Read the model definition and answer for the solid it produces. Units are mm, in the model's axes. A direction names the side the tool comes from. Round coordinates to 2 decimals unless told otherwise and drop trailing zeros. Loops run counter-clockwise (first coordinate to the right, second up) from the corner with the lowest first, then second, coordinate; pieces in that order, holes last. Notation, with made-up numbers: (31, -29.75) - (68, -29.75) arc R14 ccw to (68, -5.75) - close; hole circle Ø6 at (16, 74.5). An arc over 180 degrees is marked (long way). Use one line per item in the form item = value. Start each with the question number.
```python
from build123d import *

# Parameters (mm, degrees)
SKETCH2_W           = 33.15
SKETCH2_H           = 33
BOSS_EXTRUDE1_DEPTH = 7.5
SKETCH3_R           = 1.175
CUT_EXTRUDE1_DEPTH  = 4.5
SKETCH4_W           = 5.3
SKETCH4_H           = 7
CUT_EXTRUDE2_DEPTH  = 3.4
SKETCH5_W           = 17.312690108
SKETCH5_H           = 1.808425299
CUT_EXTRUDE3_DEPTH  = 2
SKETCH6_W           = 5.3
SKETCH6_H           = 3.3
CUT_EXTRUDE4_DEPTH  = 25.560753755
CHAMFER3_SIZE       = 11
CHAMFER3_SIZE2      = 6.350852961
SKETCH7_W           = 3
SKETCH7_H           = 33
SKETCH7_H_2         = 30
BOSS_EXTRUDE2_DEPTH = 52.5
SKETCH8_W           = 33.15
SKETCH8_H           = 60
BOSS_EXTRUDE3_DEPTH = 1
SKETCH9_W           = 3
SKETCH9_H           = 34
CUT_EXTRUDE5_DEPTH  = 60
SKETCH10_R          = 0.75
CUT_EXTRUDE6_DEPTH  = 2
SKETCH11_R          = 0.8
CUT_EXTRUDE7_DEPTH  = 2
SKETCH12_R          = 0.8
CUT_EXTRUDE9_DEPTH  = 5.8


with BuildPart() as part:
    # Sketch2 → Boss-Extrude1 (new body)
    with BuildSketch(Plane.XY):
        Rectangle(SKETCH2_W, SKETCH2_H)
    extrude(amount=BOSS_EXTRUDE1_DEPTH)

    # Sketch3 → Cut-Extrude1 (cut)
    with BuildSketch(Plane.XY):
        with Locations((10.325, 10.25)):
            Circle(SKETCH3_R)
        with Locations((-10.325, 10.25)):
            Circle(SKETCH3_R)
        with Locations((10.325, -10.25)):
            Circle(SKETCH3_R)
        with Locations((-10.325, -10.25)):
            Circle(SKETCH3_R)
    extrude(amount=CUT_EXTRUDE1_DEPTH, mode=Mode.SUBTRACT)

    # Sketch4 → Cut-Extrude2 (cut)
    with BuildSketch(Plane.XY):
        with Locations((9.775, 0)):
            Rectangle(SKETCH4_W, SKETCH4_H)
        with Locations((-9.775, 0)):
            Rectangle(SKETCH4_W, SKETCH4_H)
    extrude(amount=CUT_EXTRUDE2_DEPTH, mode=Mode.SUBTRACT)

    # Sketch5 → Cut-Extrude3 (cut)
    with BuildSketch(Plane.XY):
        with Locations((-0.109621432, -11.80915301)):
            Rectangle(SKETCH5_W, SKETCH5_H)
    extrude(amount=CUT_EXTRUDE3_DEPTH, mode=Mode.SUBTRACT)

    # Sketch6 → Cut-Extrude4 (cut, through all)
    with BuildSketch(Plane.XY):
        Rectangle(SKETCH6_W, SKETCH6_H)
    extrude(amount=CUT_EXTRUDE4_DEPTH, mode=Mode.SUBTRACT)

    # Chamfer3
    chamfer3_edges = [part.edges().sort_by_distance(p)[0] for p in [
        (2.65, 0, 7.5),
        (0, 1.65, 7.5),
        (-2.65, 0, 7.5),
        (0, -1.65, 7.5),
    ]]
    chamfer3_side = [part.faces().sort_by_distance(p)[0] for p in [
        (-16.107247662, 0, 7.5),
    ]]
    chamfer(chamfer3_edges, length=CHAMFER3_SIZE, length2=CHAMFER3_SIZE2, reference=chamfer3_side[0])

    # Sketch7 → Boss-Extrude2 (add)
    with BuildSketch(Plane.XY):
        with Locations((15.075, 0)):
            Rectangle(SKETCH7_W, SKETCH7_H)
        Polygon((-13.575, 13.5), (13.575, 13.5), (13.575, 16.5), (-16.575, 16.5), (-16.575, 13.5), align=None)
        with Locations((-15.075, -1.5)):
            Rectangle(SKETCH7_W, SKETCH7_H_2)
    extrude(amount=-BOSS_EXTRUDE2_DEPTH)

    # Sketch8 → Boss-Extrude3 (add)
    with BuildSketch(Plane(origin=(0, 16.5, 0), x_dir=(1, 0, 0), z_dir=(0, 1, 0))):
        with Locations((0, 22.5)):
            Rectangle(SKETCH8_W, SKETCH8_H)
    extrude(amount=BOSS_EXTRUDE3_DEPTH)

    # Sketch9 → Cut-Extrude5 (cut)
    with BuildSketch(Plane(origin=(0, 0, -52.5), x_dir=(-1, 0, 0), z_dir=(0, 0, -1))):
        with Locations((15.075, 0.5)):
            Rectangle(SKETCH9_W, SKETCH9_H)
    extrude(amount=-CUT_EXTRUDE5_DEPTH, mode=Mode.SUBTRACT)

    # Sketch10 → Cut-Extrude6 (cut)
    with BuildSketch(Plane.ZY.offset(13.575)):
        with Locations((-50, 15.5)):
            Circle(SKETCH10_R)
        with Locations(Location((5, 15.5, 0), (0, 0, 180))):
            Circle(SKETCH10_R)
        with Locations((5, -14.5)):
            Circle(SKETCH10_R)
    extrude(amount=-CUT_EXTRUDE6_DEPTH, mode=Mode.SUBTRACT)

    # Sketch11 → Cut-Extrude7 (cut)
    with BuildSketch(Plane(origin=(0, -16.5, 0), x_dir=(-1, 0, 0), z_dir=(0, -1, 0))):
        with Locations(Location((-15.075, 49.5, 0), (0, 0, 90))):
            Circle(SKETCH11_R)
        with Locations(Location((-15.075, -4.5, 0), (0, 0, 270))):
            Circle(SKETCH11_R)
        with Locations(Location((12.075, -4.5, 0), (0, 0, 90))):
            Circle(SKETCH11_R)
    extrude(amount=-CUT_EXTRUDE7_DEPTH, mode=Mode.SUBTRACT)

    # Sketch12 → Cut-Extrude9 (cut)
    with BuildSketch(Plane(origin=(0, 0, -52.5), x_dir=(-1, 0, 0), z_dir=(0, 0, -1))):
        with Locations((-14.575, 15.5)):
            Circle(SKETCH12_R)
        with Locations((-15.075, -14.5)):
            Circle(SKETCH12_R)
    extrude(amount=-CUT_EXTRUDE9_DEPTH, mode=Mode.SUBTRACT)


solid = part.part
```
1) Straight lines are drawn through the part: line 1 (Y direction, x = -12, z = -50); line 2 (X direction, y = -14.5, z = -48.9) (3 decimals); line 3 (Y direction, x = 6, z = -19.5). For each, find the intervals that lie inside material, in ascending order. Write a range as from..to.
2) A cutting plane is placed at D-D on y = 7.5. Write down the section's boundary in (x, z) (3 decimals), plus the area to 3 significant figures.
3) A cutting plane is placed at A-A on x = -1. Write down the section's boundary in (y, z), plus the area to 3 significant figures.
4) For faces 5 (the flat face through (10, 10, 4.5)), 6 (the flat face through (0.23, 8.3, 4.99)), 7 (the cylindrical face through (-12.589, -13.868, 5.403)), determine the directions among +Z, -Z, +X, -X, +Y, -Y from which every point of the face is accessible in a straight line to the end or side of a thin tool.
5) A cutting plane is placed at C-C on z = -41.5. Write down the section's boundary in (x, y) (3 decimals), plus the area to 3 significant figures.
6) Determine the mould class of faces 1 (the flat face through (15, -14.5, 4)), 2 (the flat face through (0.23, -8.3, 4.99)), 3 (the flat face through (15, -14, -46.7)), 4 (the flat face through (16.575, 0, -22)) for opening direction Z: +Z half, -Z half, draft (parallel to the pull), parting line (faces both ways), or undercut.
7) A cutting plane is placed at B-B on y = 0. Write down the section's boundary in (x, z) (3 decimals).
8) Flat-ended cylindrical pins translate along their axes: pin 1 (1 mm diameter, centred on x = 3.5, z = -18, fed in from -Y); pin 2 (6 mm diameter, centred on x = 1, y = 7, fed in from -Z); pin 3 (1.9 mm diameter, centred on x = 10.325, y = 10.25, fed in from +Z). Find the tip coordinate at first contact, or state that the pin passes through.
Checks:
q1.line_1 = 13.5..14.75, 16.25..17.5
q1.line_2 = 13.575..14.275, 15.875..16.575
q1.line_3 = 13.5..17.5
q2.outline = (-13.575, 0) - (13.575, 0) - (13.575, -52.5) - (16.575, -52.5) - (16.575, 7.5) - (13.65, 7.5) - (8.5, 4.527) - (-8.5, 4.527) - (-13.575, 7.457) - close
q2.area = 318 mm²
q3.outline = (-16.5, 0) - (-12.71, 0) - (-12.71, 2) - (-10.9, 2) - (-10.9, 0) - (-1.65, 0) - (-1.65, 1.15) - (-12.65, 7.5) - (-16.5, 7.5) - close; (1.65, 0) - (13.5, 0) - (13.5, -52.5) - (17.5, -52.5) - (17.5, 7.5) - (12.65, 7.5) - (1.65, 1.15) - close
q3.area = 367 mm²
q4.face_5 = -Z
q4.face_6 = +Z
q4.face_7 = -X
q5.outline = (-13.575, 13.5) - (13.575, 13.5) - (13.575, -16.5) - (16.575, -16.5) - (16.575, 17.5) - (-13.575, 17.5) - close
q5.area = 211 mm²
q6.face_1 = undercut
q6.face_2 = +Z half
q6.face_3 = -Z half
q6.face_4 = draft
q7.outline = (-13.575, 0) - (-12.425, 0) - (-12.425, 3.4) - (-7.125, 3.4) - (-7.125, 0) - (-2.65, 0) - (-2.65, 1.149) - (-13.575, 7.457) - close; (2.65, 0) - (7.125, 0) - (7.125, 3.4) - (12.425, 3.4) - (12.425, 0) - (13.575, 0) - (13.575, -52.5) - (16.575, -52.5) - (16.575, 7.5) - (13.65, 7.5) - (2.65, 1.149) - close
q8.pin_1 = 13.5
q8.pin_2 = 0
q8.pin_3 = 6.66
